Here's how the part is built. I have some questions about the finished solid (model axes, mm). A direction names the side the tool comes from. Give positions to 0.01 mm unless a question says otherwise; leave off trailing zeros. Write each loop counter-clockwise with the first axis right and the second up, starting at its lowest first coordinate (ties: lowest second). Pieces come first, ordered by that corner, then holes. Notation, with made-up numbers: (71, 87) -> (78, 87) arc R36 ccw to (78, 121) -> close; hole circle Ø7 at (-12.5, -13.75). An arc over 180 degrees is marked (long way). Use one line per item in the form item = value.
```python
from build123d import *

# Parameters (mm, degrees)
BOSS_EXTRUDE1_DEPTH      = 10
BOSS_EXTRUDE4_DEPTH      = 110
BOSS_EXTRUDE4_DEPTH_BACK = 100
SKETCH2_W                = 50.249872444
SKETCH2_H                = 9.213429789
BOSS_EXTRUDE6_DEPTH      = 210
BOSS_EXTRUDE9_DEPTH      = 70
BOSS_EXTRUDE9_DEPTH_BACK = 80
SKETCH6_W                = 38.58561731
SKETCH6_H                = 7.717123462
CUT_EXTRUDE1_DEPTH       = 70
CUT_EXTRUDE2_DEPTH       = 222.915349689
CUT_EXTRUDE2_DEPTH_BACK  = 222.915349689


with BuildPart() as part:
    # Sketch1 → Boss-Extrude1 (new body)
    with BuildSketch(Plane.XY):
        with BuildLine():
            Line((57.181832049, 10.710247908), (131.703459222, 10.710247908))
            Line((131.703459222, 10.710247908), (149.186074684, 54.392465481))
            add(Edge.make_bspline(
                [(149.186074684, 54.392465481), (168.827192519, 78.384539795), (185.224129689, 39.969217472)],
                knots=[0, 0, 0, 1, 1, 1], degree=2))
            Line((185.224129689, 39.969217472), (185.224129689, -4.90129989))
            Line((185.224129689, -4.90129989), (57.181832049, -4.90129989))
            add(Edge.make_bspline(
                [(-39.754987996, -3.086003634), (8.172307478, -26.913609431), (57.181832049, -4.90129989)],
                knots=[0, 0, 0, 1, 1, 1], degree=2))
            add(Edge.make_bspline(
                [(-47.016173018, 12.888603414), (-49.928971692, 0.460306463), (-39.754987996, -3.086003634)],
                knots=[0, 0, 0, 1, 1, 1], degree=2))
            add(Edge.make_bspline(
                [(-47.016173018, 12.888603414), (4.654032658, 48.21998755), (57.181832049, 10.710247908)],
                knots=[0, 0, 0, 1, 1, 1], degree=2))
        make_face()
    extrude(amount=BOSS_EXTRUDE1_DEPTH)

    # Sketch2 → Boss-Extrude4 (add, two sides: drawn at the far end of the back side and taken through both)
    with BuildSketch(Plane.XY.offset(-BOSS_EXTRUDE4_DEPTH_BACK)):
        with Locations((15.052306438, 4.606714895)):
            Rectangle(SKETCH2_W, SKETCH2_H)
    extrude(amount=BOSS_EXTRUDE4_DEPTH + BOSS_EXTRUDE4_DEPTH_BACK)

    # Sketch3 → Boss-Extrude6 (add)
    with BuildSketch(Plane(origin=(0, 0, -100), x_dir=(-1, 0, 0), z_dir=(0, 0, -1))):
        with BuildLine():
            Line((-40.17724266, 9.213429789), (-40.17724266, 0))
            Line((-40.17724266, 0), (10.072629784, 0))
            Line((10.072629784, 0), (10.072629784, 9.213429789))
            add(Edge.make_bspline(
                [(-40.17724266, 9.213429789), (-19.522810461, 26.526032518), (10.072629784, 9.213429789)],
                knots=[0, 0, 0, 1, 1, 1], degree=2))
        make_face()
    extrude(amount=-BOSS_EXTRUDE6_DEPTH)

    # Sketch6 → Boss-Extrude9 (add, two sides: drawn at the far end of the back side and taken through both)
    with BuildSketch(Plane.XY.offset(10).offset(-BOSS_EXTRUDE9_DEPTH_BACK)):
        with Locations((160.393476949, 6.480433212)):
            Rectangle(SKETCH6_W, SKETCH6_H)
    extrude(amount=BOSS_EXTRUDE9_DEPTH + BOSS_EXTRUDE9_DEPTH_BACK)

    # Sketch7 → Cut-Extrude1 (cut)
    with BuildSketch(Plane(origin=(0, 10.338994943, 0), x_dir=(1, 0, 0), z_dir=(0, 1, 0))):
        with BuildLine():
            Line((141.100668294, -10), (141.100668294, -80))
            Line((141.100668294, -80), (155.374228958, -80))
            add(Edge.make_bspline(
                [(141.100668294, -10), (141.156131379, -46.554762938), (155.374228958, -80)],
                knots=[0, 0, 0, 1, 1, 1], degree=2))
        make_face()
    extrude(amount=-CUT_EXTRUDE1_DEPTH, mode=Mode.SUBTRACT)

    # Sketch10 → Cut-Extrude2 (cut, two sides: drawn at the far end of the back side and taken through both)
    with BuildSketch(Plane(origin=(0, 10.338994943, 0), x_dir=(1, 0, 0), z_dir=(0, 1, 0)).offset(-CUT_EXTRUDE2_DEPTH_BACK)):
        with BuildLine():
            Line((141.100668294, 70), (141.100668294, 0))
            add(Edge.make_bspline(
                [(141.100668294, 0), (144.11108971, 35.90170366), (155.374228958, 70)],
                knots=[0, 0, 0, 1, 1, 1], degree=2))
            Line((155.374228958, 70), (141.100668294, 70))
        make_face()
    extrude(amount=CUT_EXTRUDE2_DEPTH + CUT_EXTRUDE2_DEPTH_BACK, mode=Mode.SUBTRACT)


solid = part.part
```
Q1. I want a section at A-A, the plane x = 125.5. Write out the boundary of the cut face in (y, z).
Result set:
outline = (-4.9, 0) -> (10.71, 0) -> (10.71, 10) -> (-4.9, 10) -> close
Q2. If we mould it in two halves opening along X, with no side actions, what happens to faces 5 (the face through (15, 0, 59)), 6 (the face through (185.224, 18, 5)), 7 (the face through (40.177, 5, 59)), 8 (the face through (40.177, 5, -51))? For each: +X half, -X half, draft (parallel to the pull), parting line (faces both ways), or undercut.
Result set:
face_5 = draft
face_6 = +X half
face_7 = undercut
face_8 = undercut
Q3. Which directions (+Z, -Z, +X, -X, +Y, -Y) give clear straight access to the entire face, cutting with the end or side of a thin tool? Please do faces 1 (the face through (122, -4.901, 5)), 2 (the face through (15, 0, -51)), 3 (the face through (94, 10.71, 5)), 4 (the face through (160, 10.339, 45)).
Result set:
face_1 = +Z, -Z, +X, -Y
face_2 = -Z, +X, -X, -Y
face_3 = +Z, -Z, +Y
face_4 = +Z, +X, +Y
Q4. If I drill on line 1 along Z through (x, y) = (28, -9); line 2 along X through (y, z) = (8.5, -6); line 3 along X through (y, z) = (9, -66.5), over which ranges is the centre line in solid material (lowest first)? Write a range as from..to.
Result set:
line_1 = 0..10
line_2 = -10.07..40.18, 141.66..179.69
line_3 = -10.07..40.18, 154.24..179.69
Q5. Will these pins go through, and if not, where does the flat tip stop? pin 1 Ø3 at (y, z) = (6, 79.5) entering from +X; pin 2 Ø11.5 at (x, z) = (165.5, -25) entering from -Y; pin 3 Ø23.5 at (x, y) = (105.5, 31) entering from -Z; pin 4 Ø1.5 at (x, y) = (126, 3.5) entering from -Z.
Result set:
pin_1 = 179.69
pin_2 = 2.62
pin_3 = through
pin_4 = 0
